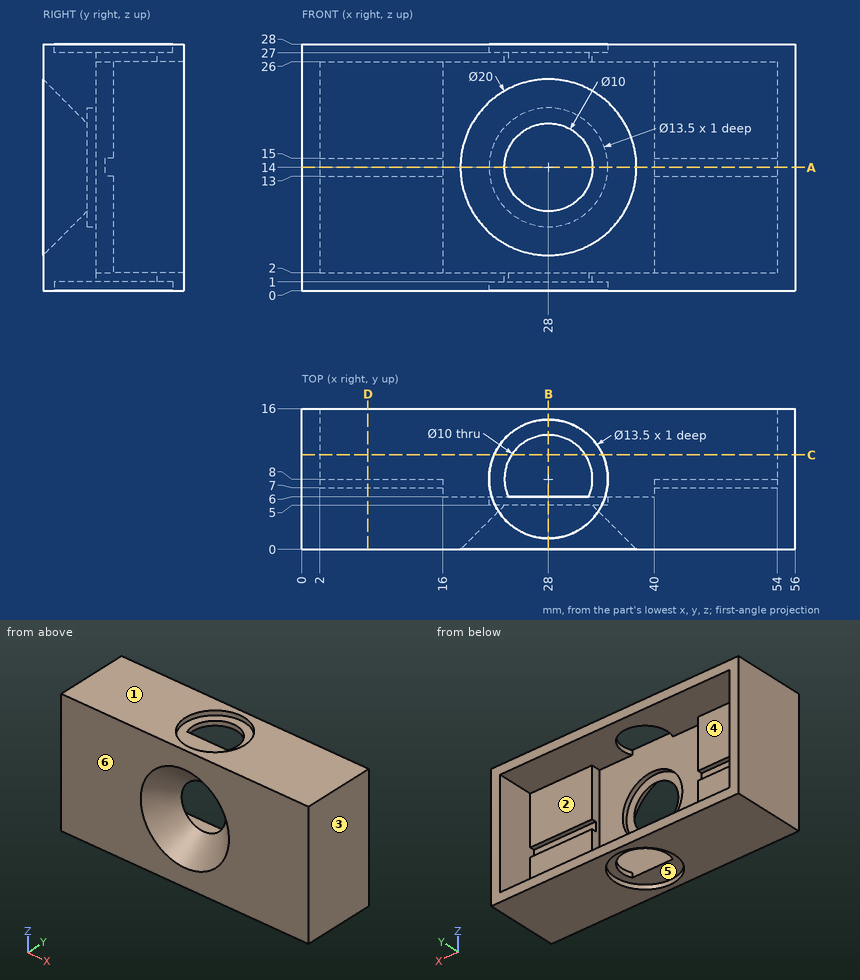
Source: three-view drawing plus pictorial views. Frame: mm from the lowest corner of the part. A direction names the side the tool comes from. Give positions to 0.01 mm unless a question says otherwise; leave off trailing zeros. Order: outer loops, then holes, each group sorted by start corner. A loop starts at its lowest first (then second) coordinate and runs counter-clockwise, first axis right, second up.
1. Material intervals for L1, parallel to Y at x = 28, z = 26.85; L2, parallel to Z at x = 40.5, y = 14; L3, parallel to Y at x = 28, z = 0.45, sorted ascending.
Derived:
L1: y = 0 to 6, 13 to 16
L2: z = 0 to 2, 26 to 28
L3: y = 0 to 1.25, 14.75 to 16
2. Pin query (flat end, axial travel): pin 1 (11 mm diameter, centred on x = 29, z = 12.5, fed in from +Y); pin 2 (2 mm diameter, centred on x = 23.5, y = 6.5, fed in from -Z); pin 3 (5.5 mm diameter, centred on x = 44.5, z = 23, fed in from +Y). Return the tip coordinate at first contact, or that it passes through.
Derived:
pin 1: stops at y = 6
pin 2: stops at z = 1
pin 3: stops at y = 8
3. Section B-B on x = 28. Return the cut outline in (y, z), and give its area (3 significant figures).
Derived:
outline: (0, 0) - (1.25, 0) - (1.25, 1) - (6, 1) - (6, 7.25) - (5, 7.25) - (5, 9) - (0, 4) - close; (0, 24) - (5, 19) - (5, 20.75) - (6, 20.75) - (6, 27) - (1.25, 27) - (1.25, 28) - (0, 28) - close; (13, 1) - (14.75, 1) - (14.75, 0) - (16, 0) - (16, 2) - (13, 2) - close; (13, 26) - (16, 26) - (16, 28) - (14.75, 28) - (14.75, 27) - (13, 27) - close
area: 78.5 mm2
4. Section C-C on y = 10.75. Return the cut outline in (x, z), and give its area (3 significant figures).
Derived:
outline: (0, 0) - (21.84, 0) - (21.84, 1) - (23.82, 1) - (23.82, 2) - (2, 2) - (2, 26) - (23.82, 26) - (23.82, 27) - (21.84, 27) - (21.84, 28) - (0, 28) - close; (32.18, 1) - (34.16, 1) - (34.16, 0) - (56, 0) - (56, 28) - (34.16, 28) - (34.16, 27) - (32.18, 27) - (32.18, 26) - (54, 26) - (54, 2) - (32.18, 2) - close
area: 279 mm2
5. Section A-A on z = 14. Return the cut outline in (x, y).
Derived:
outline: (0, 0) - (18, 0) - (23, 5) - (21.25, 5) - (21.25, 6) - (16, 6) - (16, 7) - (2, 7) - (2, 16) - (0, 16) - close; (33, 5) - (38, 0) - (56, 0) - (56, 16) - (54, 16) - (54, 7) - (40, 7) - (40, 6) - (34.75, 6) - (34.75, 5) - close
6. Mould query, pull axis Z, two halves, no side actions, for the marked faces 1, 2 and 3. Classes: released by +Z, released by -Z, zero draft, split by the parting line, or undercut.
Derived:
face 1: released by +Z
face 2: undercut
face 3: zero draft
7. Section D-D on x = 7.5. Return the cut outline in (y, z), and give its area (3 significant figures).
Derived:
outline: (0, 0) - (16, 0) - (16, 2) - (8, 2) - (8, 13) - (7, 13) - (7, 15) - (8, 15) - (8, 26) - (16, 26) - (16, 28) - (0, 28) - close
area: 254 mm2
8. Reachability of the marked faces 4, 5 and 6 from +Z, -Z, +X, -X, +Y, -Y: full face, straight path, thin tool, end or side. Return the list, or none.
Derived:
face 4: +Y
face 5: -Z
face 6: +Z, -Z, +X, -X, -Y
